Design review of the part built by this model. Coordinates are the model's own, in mm. Face numbers are marked on the shaded views. A direction names the side the tool comes from. Give positions to 0.01 mm unless a question says otherwise; leave off trailing zeros. Write each loop counter-clockwise with the first axis right and the second up, starting at its lowest first coordinate (ties: lowest second). Pieces come first, ordered by that corner, then holes. Notation, with made-up numbers: (-3.5, 22.25) -> (6.5, 22.25) arc R28 ccw to (6.5, 45.25) -> close; hole circle Ø7 at (-40, -27.75). An arc over 180 degrees is marked (long way). Return JSON: item names as keys, results as strings. Group by question number.
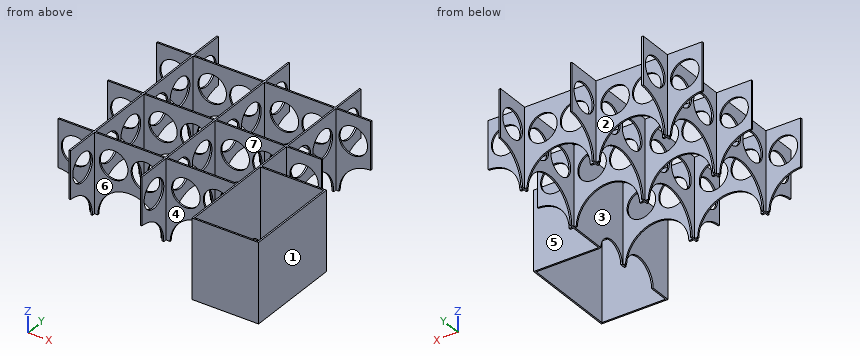
from build123d import *

# Parameters (mm, degrees)
F0_W      = 1
F0_H      = 22
F0_W_2    = 22
F0_H_2    = 1
F0_W_3    = 44
F0_H_3    = 44
F0_H_4    = 23
F1_DEPTH  = 50
F2_R      = 9
F3_DEPTH  = 500
F4_R      = 9
F5_DEPTH  = 500
F6_R      = 9
F7_DEPTH  = 500
F8_R      = 9
F9_DEPTH  = 500
F10_R     = 9
F11_DEPTH = 500
F12_R     = 9
F13_DEPTH = 500
F14_R     = 9
F15_DEPTH = 500
F16_R     = 9
F17_DEPTH = 400
F18_R     = 12.5
F19_DEPTH = 1


with BuildPart() as f1:
    # F0 (on Top) → F1 (new body)
    with BuildSketch(Plane.XY):
        with Locations((-45, 56.5)):
            Rectangle(F0_W, F0_H)
        with Locations((-56.5, 45)):
            Rectangle(F0_W_2, F0_H_2)
        with Locations((-22.5, 45)):
            Rectangle(F0_W_3, F0_H_2)
        with Locations((-45, 22.5)):
            Rectangle(F0_W, F0_H_3)
        with Locations((-45, 45)):
            Rectangle(F0_W, F0_H_2)
        with Locations((0, 56.5)):
            Rectangle(F0_W, F0_H)
        Polygon((0.5, 45.5), (0.5, 44.5), (44.5, 44.5), (45.5, 44.5), (67.5, 44.5), (67.5, 45.5), (45.5, 45.5), (44.5, 45.5), align=None)
        with Locations((45, 56.5)):
            Rectangle(F0_W, F0_H)
        with Locations((0, 45)):
            Rectangle(F0_W, F0_H_2)
        with Locations((0, 22.5)):
            Rectangle(F0_W, F0_H_3)
        with Locations((45, 22.5)):
            Rectangle(F0_W, F0_H_3)
        Polygon((0.5, 0.5), (0.5, -0.5), (44.5, -0.5), (45.5, -0.5), (67.5, -0.5), (67.5, 0.5), (45.5, 0.5), (44.5, 0.5), align=None)
        with Locations((45, -12)):
            Rectangle(F0_W, F0_H_4)
        Rectangle(F0_W, F0_H_2)
        with Locations((-22.5, 0)):
            Rectangle(F0_W_3, F0_H_2)
        with Locations((0, -22.5)):
            Rectangle(F0_W, F0_H_3)
        with Locations((-56.5, 0)):
            Rectangle(F0_W_2, F0_H_2)
        with Locations((-45, -22.5)):
            Rectangle(F0_W, F0_H_3)
        with Locations((-45, 0)):
            Rectangle(F0_W, F0_H_2)
        with Locations((-56.5, -45)):
            Rectangle(F0_W_2, F0_H_2)
        with Locations((-45, -56.5)):
            Rectangle(F0_W, F0_H)
        with Locations((-45, -45)):
            Rectangle(F0_W, F0_H_2)
        with Locations((-22.5, -45)):
            Rectangle(F0_W_3, F0_H_2)
        with Locations((0, -56.5)):
            Rectangle(F0_W, F0_H)
        with Locations((22.5, -45)):
            Rectangle(F0_W_3, F0_H_2)
        with Locations((0, -45)):
            Rectangle(F0_W, F0_H_2)
        Polygon((44.5, -44.5), (44.5, -45.5), (44.5, -85.5), (86.5, -85.5), (86.5, -23.5), (45.5, -23.5), (44.5, -23.5), align=None)
        Polygon((45.5, -45.4983576005), (45.5, -44.4983576005), (45.5, -24.5), (85.5, -24.5), (85.5, -84.5), (45.5, -84.5), align=None, mode=Mode.SUBTRACT)
    extrude(amount=F1_DEPTH)

    # F2 (on face) → F3 (cut)
    with BuildSketch(Plane.XZ.offset(45.5)):
        with Locations((-32.5, 34)):
            Circle(F2_R)
        with Locations((-12.5, 34)):
            Circle(F2_R)
        with BuildLine():
            Line((-42.5, 0), (-2.5, 0))
            ThreePointArc((-2.5, 0), (-22.5, 20), (-42.5, 0))
        make_face()
    extrude(amount=-F3_DEPTH, mode=Mode.SUBTRACT)

    # F4 (on face) → F5 (cut)
    with BuildSketch(Plane.XZ.offset(45.5)):
        with Locations((13.0384618044, 33.2217942973)):
            Circle(F4_R)
        with Locations((33.0384618044, 33.2217942973)):
            Circle(F4_R)
        with BuildLine():
            Line((3.0536076422, 0), (43.0233159666, 0))
            ThreePointArc((43.0233159666, 0), (23.0384618044, 19.2217942973), (3.0536076422, 0))
        make_face()
    extrude(amount=-F5_DEPTH, mode=Mode.SUBTRACT)

    # F6 (on face) → F7 (cut)
    with BuildSketch(Plane.XZ.offset(45.5)):
        with Locations((-56.5, 34)):
            Circle(F6_R)
        with BuildLine():
            ThreePointArc((-67.5, 20), (-81.6421356237, -14.1421356237), (-47.5, 0))
            ThreePointArc((-47.5, 0), (-53.3578643763, 14.1421356237), (-67.5, 20))
        make_face()
    extrude(amount=-F7_DEPTH, mode=Mode.SUBTRACT)

    # F8 (on face) → F9 (cut)
    with BuildSketch(Plane.YZ.offset(0.5)):
        with Locations((-12.5, 34)):
            Circle(F8_R)
        with BuildLine():
            Line((-42.5, 0), (-2.5, 0))
            ThreePointArc((-2.5, 0), (-22.5, 20), (-42.5, 0))
        make_face()
        with Locations((-32.5, 34)):
            Circle(F8_R)
    extrude(amount=-F9_DEPTH, mode=Mode.SUBTRACT)

    # F10 (on face) → F11 (cut)
    with BuildSketch(Plane.YZ.offset(0.5)):
        with Locations((-56.5, 34)):
            Circle(F10_R)
        with BuildLine():
            Line((-67.5, 0), (-47.5, 0))
            ThreePointArc((-47.5, 0), (-53.3578643763, 14.1421356237), (-67.5, 20))
            Line((-67.5, 20), (-67.5, 0))
        make_face()
    extrude(amount=-F11_DEPTH, mode=Mode.SUBTRACT)

    # F12 (on face) → F13 (cut)
    with BuildSketch(Plane.YZ.offset(45.5)):
        with Locations((12.5, 34)):
            Circle(F12_R)
        with Locations((32.5, 34)):
            Circle(F12_R)
        with BuildLine():
            Line((2.5, 0), (42.5, 0))
            ThreePointArc((42.5, 0), (22.5, 20), (2.5, 0))
        make_face()
    extrude(amount=-F13_DEPTH, mode=Mode.SUBTRACT)

    # F14 (on face) → F15 (cut)
    with BuildSketch(Plane.YZ.offset(45.5)):
        with BuildLine():
            Line((67.5, 0), (67.5, 20))
            ThreePointArc((67.5, 20), (53.3578643763, 14.1421356237), (47.5, 0))
            Line((47.5, 0), (67.5, 0))
        make_face()
        with Locations((56.5, 34)):
            Circle(F14_R)
    extrude(amount=-F15_DEPTH, mode=Mode.SUBTRACT)

    # F16 (on face) → F17 (cut)
    with BuildSketch(Plane.XZ.offset(0.5)):
        with Locations((56.5, 34)):
            Circle(F16_R)
        with BuildLine():
            Line((67.5, 0), (67.5, 20))
            ThreePointArc((67.5, 20), (53.3578643763, 14.1421356237), (47.5, 0))
            Line((47.5, 0), (67.5, 0))
        make_face()
    extrude(amount=-F17_DEPTH, mode=Mode.SUBTRACT)

    # F18 (on face) → F19 (cut)
    with BuildSketch(Plane(origin=(44.5, 0, 0), x_dir=(0, -1, 0), z_dir=(-1, 0, 0))):
        with BuildLine():
            Line((24.25, 0), (43.75, 0))
            ThreePointArc((43.75, 0), (34, 9.75), (24.25, 0))
        make_face()
        with Locations((59.5, 0)):
            Circle(F18_R)
    extrude(amount=-F19_DEPTH, mode=Mode.SUBTRACT)


solid = f1.part
Q1. Mouldability with a two-part tool opening along Y and no side actions: class the marked faces 1, 2, 3 and 4 as +Y half, -Y half, draft (parallel to the pull), parting line (faces both ways), or undercut.
Q2. Take a section at C-C, the plane y = -57. Give the boundary of the cut face in (x, z), plus the area to 3 significant figures.
Q3. For L1, parallel to X at y = -27, z = 43; L2, parallel to Y at x = -8, z = 22.5, list the stretches that pass through material, from the lowest coordinate up. Write a range as from..to.
Q4. Take a section at A-A, the plane y = -75. Give the boundary of the cut face in (x, z), plus the area to 3 significant figures.
Q5. Tool access review of the marked faces 5, 6 and 7: name each direction out of +Z, -Z, +X, -X, +Y, -Y from which nothing blocks a thin tool from reaching the whole face with its end or side.
Q6. Take a section at B-B, the plane x = -56.5. Give the boundary of the cut face in (y, z).
Q7. Take a section at D-D, the plane y = -18. Give the boundary of the cut face in (x, z), plus the area to 3 significant figures.
Q8. Insertion check: pin 1 (6 mm diameter, centred on y = 7.5, z = 32, fed in from +X); pin 2 (20.5 mm diameter, centred on x = 33.04, z = 33.22, fed in from +Y); pin 3 (5 mm diameter, centred on y = 1.5, z = 27.5, fed in from +X); pin 4 (1 mm diameter, centred on y = -33.5, z = 16, fed in from -X). Each pin has a flat end and moves straight along its axis. Give the tip position at first contact, or say it passes through.
Final values:
{
 "1": {"face 1": "draft", "face 2": "+Y half", "face 3": "undercut", "face 4": "-Y half"},
 "2": {"outline": "(-45.5, 17.02) -> (-44.5, 17.02) -> (-44.5, 25.01) -> (-45.5, 25.01) -> close; (-45.5, 42.99) -> (-44.5, 42.99) -> (-44.5, 50) -> (-45.5, 50) -> close; (-0.5, 17.02) -> (0.5, 17.02) -> (0.5, 25.01) -> (-0.5, 25.01) -> close; (-0.5, 42.99) -> (0.5, 42.99) -> (0.5, 50) -> (-0.5, 50) -> close; (44.5, 12.25) -> (45.5, 12.25) -> (45.5, 50) -> (44.5, 50) -> close; (85.5, 0) -> (86.5, 0) -> (86.5, 50) -> (85.5, 50) -> close", "area": "118 mm²"},
 "3": {"L1": "x = -45.5..-44.5, -0.5..0.5, 44.5..45.5, 85.5..86.5", "L2": "y = -45.5..-44.5, -0.5..0.5, 44.5..45.5"},
 "4": {"outline": "(44.5, 0) -> (45.5, 0) -> (45.5, 50) -> (44.5, 50) -> close; (85.5, 0) -> (86.5, 0) -> (86.5, 50) -> (85.5, 50) -> close", "area": "100 mm²"},
 "5": {"face 5": "+Z, -Z, +X", "face 6": "+Z, -Z, -Y", "face 7": "+Z, -Z"},
 "6": {"outline": "(-45.5, 16.7) -> (-44.5, 16.7) -> (-44.5, 25) -> (-45.5, 25) -> close; (-45.5, 43) -> (-44.5, 43) -> (-44.5, 50) -> (-45.5, 50) -> close; (-0.5, 16.7) -> (0.5, 16.7) -> (0.5, 25) -> (-0.5, 25) -> close; (-0.5, 43) -> (0.5, 43) -> (0.5, 50) -> (-0.5, 50) -> close; (44.5, 16.7) -> (45.5, 16.7) -> (45.5, 25) -> (44.5, 25) -> close; (44.5, 43) -> (45.5, 43) -> (45.5, 50) -> (44.5, 50) -> close"},
 "7": {"outline": "(-45.5, 19.49) -> (-44.5, 19.49) -> (-44.5, 26.88) -> (-45.5, 26.88) -> close; (-45.5, 41.12) -> (-44.5, 41.12) -> (-44.5, 50) -> (-45.5, 50) -> close; (-0.5, 19.49) -> (0.5, 19.49) -> (0.5, 26.88) -> (-0.5, 26.88) -> close; (-0.5, 41.12) -> (0.5, 41.12) -> (0.5, 50) -> (-0.5, 50) -> close; (44.5, 0) -> (45.5, 0) -> (45.5, 50) -> (44.5, 50) -> close", "area": "82.5 mm²"},
 "8": {"pin 1": "passes through", "pin 2": "stops at y = 45.5", "pin 3": "stops at x = 67.5", "pin 4": "stops at x = 44.5"}
}
